Work out the finished part from the listing and answer in its coordinate system (mm). A direction names the side the tool comes from. Coordinates: 2 decimals unless noted, no trailing zeros. Order: outer loops, then holes, each group sorted by start corner. A loop starts at its lowest first (then second) coordinate and runs counter-clockwise, first axis right, second up. Notation, with made-up numbers: M 63.5,37.5 L 92.5,37.5 A21 ccw 92.5,41.5 Z; hole C 56,-17 d8. An arc over 180 degrees is marked long. Answer in a Markdown table with one row per item. Add a question column.
Item 1: The mould has two halves that part along X. Classify faces 1 (the face through (95, 5, 1)), 2 (the face through (-30.53, 2.46, 25.46)), 3 (the face through (-41, 5, -1)): released by +X, released by -X, zero draft, split by the parting line, or undercut.
Item 2: The part is cut by section C-C (y = 8.5). State how many separate pieces and enclosed holes the cut face has, then the cut area to 3 significant figures.
Item 3: The part is cut by section D-D (z = 25). Write down the section's boundary in (x, y), then the cut area to 3 significant figures.
Item 4: The part is cut by section A-A (z = -30.4). Write down the section's boundary in (x, y), then the cut area to 3 significant figures.
Item 5: Consider line 1 (X direction, y = 5.25, z = -21); line 2 (X direction, y = 4.5, z = 34); line 3 (X direction, y = 8.1, z = -30.4). Determine where each line is inside the solid, lowest interval first. Write a range as from..to.
Item 6: Flat-ended cylindrical pins translate along their axes: pin 1 Ø9 at (x, z) = (-84, 25) entering from +Y; pin 2 Ø1.5 at (y, z) = (6.5, -14.5) entering from -X. Find the tip coordinate at first contact, or state that the pin passes through.
Item 7: Which of the six approach directions +Z, -Z, +X, -X, +Y, -Y give full straight-line access (tool end or side, diameter ignored) to faces 4 (the face through (-87.417, 2.465, -24.241)), 5 (the face through (91.298, 3.451, -30.202))?
Item 8: The part is cut by section B-B (x = 66.5). Write down the section's boundary in (y, z), then the cut area to 3 significant figures.
from build123d import *

# Parameters (mm, degrees)
SKETCH1_W           = 190
SKETCH1_H           = 80
BOSS_EXTRUDE1_DEPTH = 5
SKETCH3_W           = 80
SKETCH3_H           = 80
BOSS_EXTRUDE2_DEPTH = 5
SKETCH4_R           = 1.55
CUT_EXTRUDE1_DEPTH  = 104.561575886
SKETCH5_R           = 6.5
CUT_EXTRUDE2_DEPTH  = 104.561575886
CUT_EXTRUDE3_DEPTH  = 7
SKETCH7_R           = 3.5
CUT_EXTRUDE4_DEPTH  = 104.561575886


with BuildPart() as part:
    # Sketch1 → Boss-Extrude1 (new body)
    with BuildSketch(Plane(origin=(0, 0, 0), x_dir=(1, 0, 0), z_dir=(0, 1, 0))):
        Rectangle(SKETCH1_W, SKETCH1_H)
    extrude(amount=BOSS_EXTRUDE1_DEPTH)

    # Sketch3 → Boss-Extrude2 (add)
    with BuildSketch(Plane(origin=(0, 5, 0), x_dir=(1, 0, 0), z_dir=(0, 1, 0))):
        with Locations((55, 0)):
            Rectangle(SKETCH3_W, SKETCH3_H)
    extrude(amount=BOSS_EXTRUDE2_DEPTH)

    # Sketch4 → Cut-Extrude1 (cut, through all)
    with BuildSketch(Plane(origin=(0, 10, 0), x_dir=(1, 0, 0), z_dir=(0, 1, 0))):
        with Locations(Location((22, 21, 0), (0, 0, 270))):
            Circle(SKETCH4_R)
        with Locations(Location((89, 21, 0), (0, 0, 270))):
            Circle(SKETCH4_R)
        with Locations(Location((22, -34, 0), (0, 0, 270))):
            Circle(SKETCH4_R)
        with Locations(Location((89, -34, 0), (0, 0, 270))):
            Circle(SKETCH4_R)
    extrude(amount=-CUT_EXTRUDE1_DEPTH, mode=Mode.SUBTRACT)

    # Sketch5 → Cut-Extrude2 (cut, through all)
    with BuildSketch(Plane.XZ):
        with Locations(Location((31.4, -30.4, 0), (0, 0, 270))):
            Circle(SKETCH5_R)
        with Locations(Location((47.2, -30.4, 0), (0, 0, 270))):
            Circle(SKETCH5_R)
        with Locations(Location((66.5, -30.4, 0), (0, 0, 270))):
            Circle(SKETCH5_R)
        with Locations(Location((82.3, -30.4, 0), (0, 0, 270))):
            Circle(SKETCH5_R)
    extrude(amount=-CUT_EXTRUDE2_DEPTH, mode=Mode.SUBTRACT)

    # Sketch6 → Cut-Extrude3 (cut)
    with BuildSketch(Plane.XZ):
        with BuildLine():
            Line((31.4, -21.4), (82.3, -21.4))
            ThreePointArc((82.3, -21.4), (91.3, -30.4), (82.3, -39.4))
            Line((82.3, -39.4), (31.4, -39.4))
            ThreePointArc((31.4, -39.4), (22.4, -30.4), (31.4, -21.4))
        make_face()
    extrude(amount=-CUT_EXTRUDE3_DEPTH, mode=Mode.SUBTRACT)

    # Sketch7 → Cut-Extrude4 (cut, through all)
    with BuildSketch(Plane.XZ):
        with Locations(Location((-84, 25, 0), (0, 0, 270))):
            Circle(SKETCH7_R)
        with Locations(Location((-34, 25, 0), (0, 0, 270))):
            Circle(SKETCH7_R)
        with Locations(Location((-84, -25, 0), (0, 0, 270))):
            Circle(SKETCH7_R)
        with Locations(Location((-34, -25, 0), (0, 0, 270))):
            Circle(SKETCH7_R)
    extrude(amount=-CUT_EXTRUDE4_DEPTH, mode=Mode.SUBTRACT)


solid = part.part
Reply:
| question | item | result |
|---|---|---|
| 1 | face 1 | released by +X |
| 1 | face 2 | undercut |
| 1 | face 3 | zero draft |
| 2 | separate pieces | 1 |
| 2 | enclosed holes | 8 |
| 2 | area | 5,840 mm2 |
| 3 | outline | M -95,0 L -87.5,0 L -87.5,5 L -95,5 Z; M -80.5,0 L -37.5,0 L -37.5,5 L -80.5,5 Z; M -30.5,0 L 95,0 L 95,10 L 15,10 L 15,5 L -30.5,5 Z |
| 3 | area | 1,280 mm2 |
| 4 | outline | M -95,0 L 22.4,0 L 22.4,7 L 24.9,7 L 24.9,10 L 15,10 L 15,5 L -95,5 Z; M 37.9,7 L 40.7,7 L 40.7,10 L 37.9,10 Z; M 53.7,7 L 60,7 L 60,10 L 53.7,10 Z; M 73,7 L 75.8,7 L 75.8,10 L 73,10 Z; M 88.8,7 L 91.3,7 L 91.3,0 L 95,0 L 95,10 L 88.8,10 Z |
| 4 | area | 712 mm2 |
| 5 | line 1 | x = 15..20.45, 23.55..87.45, 90.55..95 |
| 5 | line 2 | x = -95..20.45, 23.55..87.45, 90.55..95 |
| 5 | line 3 | x = 15..24.9, 37.9..40.7, 53.7..60, 73..75.8, 88.8..95 |
| 6 | pin 1 | stops at y = 5 |
| 6 | pin 2 | stops at x = 15 |
| 7 | face 4 | +Y, -Y |
| 7 | face 5 | -Y |
| 8 | outline | M 0,-40 L 10,-40 L 10,-36.9 L 7,-36.9 L 7,-39.4 L 0,-39.4 Z; M 0,-21.4 L 7,-21.4 L 7,-23.9 L 10,-23.9 L 10,40 L 0,40 Z |
| 8 | area | 635 mm2 |
